Read the model definition and answer for the solid it produces. Units are mm, in the model's axes. A direction names the side the tool comes from. Coordinates: 2 decimals unless noted, no trailing zeros. Loops run counter-clockwise (first coordinate to the right, second up) from the corner with the lowest first, then second, coordinate; pieces in that order, holes last.
from build123d import *

# Parameters (mm, degrees)
F0_W     = 92.0124906
F0_H     = 21.3499954
F0_R     = 6.7062477
F1_DEPTH = 1.5875
F2_R     = 10.6749977
F4_DEPTH = 12
F5_R     = 2.2479
F6_DEPTH = 13.5875
F7_R     = 3.96875
F8_DEPTH = 7.2375014


with BuildPart() as f1:
    # F0 (on Top) → F1 (new body)
    with BuildSketch(Plane.XY):
        with Locations((46.0062453, -10.6749977)):
            Rectangle(F0_W, F0_H)
        with Locations((10.6749977, -10.6749977)):
            Circle(F0_R, mode=Mode.SUBTRACT)
        with Locations((81.3374929, -10.6749977)):
            Circle(F0_R, mode=Mode.SUBTRACT)
    extrude(amount=F1_DEPTH)

    # F2
    f2_edges = [f1.edges().sort_by_distance(p)[0] for p in [
        (0, 0, 0.79375),
        (92.012491, 0, 0.79375),
    ]]
    fillet(f2_edges, radius=F2_R)

    # F3 (on face) → F4 (join)
    with BuildSketch(Plane.XY.offset(1.5875)):
        with BuildLine():
            Line((4.5476495872, -14.9999954), (0, -14.9999954))
            Line((0, -14.9999954), (0, -21.3499954))
            Line((0, -21.3499954), (92.0124906, -21.3499954))
            Line((92.0124906, -21.3499954), (92.0124906, -14.9999954))
            Line((92.0124906, -14.9999954), (87.4648410128, -14.9999954))
            ThreePointArc((87.4648410128, -14.9999954), (81.3374929, -18.1749977), (75.2101447872, -14.9999954))
            Line((75.2101447872, -14.9999954), (16.8023458128, -14.9999954))
            ThreePointArc((16.8023458128, -14.9999954), (10.6749977, -18.1749977), (4.5476495872, -14.9999954))
        make_face()
        with BuildLine():
            Line((0, -10.6749977), (0, -14.9999954))
            Line((0, -14.9999954), (4.5476495872, -14.9999954))
            ThreePointArc((4.5476495872, -14.9999954), (8.4061996532, -3.5263925617), (18.1749977, -10.6749977))
            ThreePointArc((18.1749977, -10.6749977), (17.8236028383, -12.9437957468), (16.8023458128, -14.9999954))
            Line((16.8023458128, -14.9999954), (75.2101447872, -14.9999954))
            ThreePointArc((75.2101447872, -14.9999954), (79.0686948532, -3.5263925617), (88.8374929, -10.6749977))
            ThreePointArc((88.8374929, -10.6749977), (88.4860980383, -12.9437957468), (87.4648410128, -14.9999954))
            Line((87.4648410128, -14.9999954), (92.0124906, -14.9999954))
            Line((92.0124906, -14.9999954), (92.0124906, -10.6749977))
            ThreePointArc((92.0124906, -10.6749977), (88.8858561628, -3.1266344372), (81.3374929, 0))
            Line((81.3374929, 0), (10.6749977, 0))
            ThreePointArc((10.6749977, 0), (3.1266344372, -3.1266344372), (0, -10.6749977))
        make_face()
    extrude(amount=F4_DEPTH)

    # F5 (on face) → F6 (cut, through all)
    with BuildSketch(Plane.XY.offset(13.5875)):
        with Locations((25.3187477, -10.6749977)):
            Circle(F5_R)
        with Locations((66.6937429, -10.6749977)):
            Circle(F5_R)
        with BuildLine():
            ThreePointArc((46.0062453, -10.8706539), (48.2513093303, -9.9407179303), (49.1812453, -7.6956539))
            ThreePointArc((49.1812453, -7.6956539), (43.7611812697, -5.4505898697), (46.0062453, -10.8706539))
        make_face()
    extrude(amount=-F6_DEPTH, mode=Mode.SUBTRACT)

    # F7 (on face) → F8 (cut)
    with BuildSketch(Plane(origin=(0, 0, 0), x_dir=(1, 0, 0), z_dir=(0, 0, -1))):
        with Locations((66.6937429, 10.6749977)):
            Circle(F7_R)
        with Locations((25.3187477, 10.6749977)):
            Circle(F7_R)
    extrude(amount=-F8_DEPTH, mode=Mode.SUBTRACT)


solid = f1.part
Q1. Which of the six approach directions +Z, -Z, +X, -X, +Y, -Y give full straight-line access (tool end or side, diameter ignored) to faces 4 (the face through (68.4, -8.97, 7.238)), 5 (the face through (47, 0, 7)), 6 (the face through (5, -15, 1.588))?
Findings below:
face 4: -Z
face 5: +Z, -Z, +X, -X, +Y
face 6: +Z
Q2. A cutting plane is placed at D-D (x = 85). Give the vertices of the cut face in (y, z), then the cut area to 3 significant figures.
Findings below:
outline: (-21.35, 0) - (-16.29, 0) - (-16.29, 1.59) - (-17.22, 1.59) - (-17.22, 13.59) - (-21.35, 13.59) - close; (-5.06, 0) - (-0.65, 0) - (-0.65, 13.59) - (-4.13, 13.59) - (-4.13, 1.59) - (-5.06, 1.59) - close
area: 106 mm2
Q3. A cutting plane is placed at A-A (z = 3.5). Count the separate pieces of the cut face and the enclosed holes in it, then the cut area to 3 significant figures.
Findings below:
separate pieces: 1
enclosed holes: 5
area: 1,430 mm2
Q4. Determine the mould class of faces 1 (the face through (63.544, -8.26, 3.568)), 2 (the face through (45, -21.35, 7)), 3 (the face through (92.012, -16, 7)) for opening direction Y: +Y half, -Y half, draft (parallel to the pull), parting line (faces both ways), or undercut.
Findings below:
face 1: undercut
face 2: -Y half
face 3: draft
Q5. Flat-ended cylindrical pins translate along their axes: pin 1 Ø7 at (x, y) = (66.69, -10.67) entering from -Z; pin 2 Ø12 at (x, y) = (65, -14.5) entering from -Z; pin 3 Ø6 at (y, z) = (-5, 7.5) entering from -X. Find the tip coordinate at first contact, or state that the pin passes through.
Findings below:
pin 1: stops at z = 7.24
pin 2: stops at z = 0
pin 3: stops at x = 0.34
Q6. Straight lines are drawn through the part: probe 1 along X at (y, z) = (-7.75, 2); probe 2 along X at (y, z) = (-6, 13.25); probe 3 along X at (y, z) = (-15.25, 4). For each, find the intervals that lie inside material, in ascending order.
Findings below:
probe 1: x = 0.41 to 3.77, 17.58 to 22.64, 28 to 42.83, 49.18 to 64.01, 69.38 to 74.43, 88.24 to 91.6
probe 2: x = 1.08 to 4.81, 16.54 to 43.32, 48.69 to 75.47, 87.2 to 90.93
probe 3: x = 0 to 4.73, 16.62 to 75.39, 87.28 to 92.01
Q7. A cutting plane is placed at B-B (x = 47.5). Give the vertices of the cut face in (y, z).
Findings below:
outline: (-21.35, 0) - (-10.5, 0) - (-10.5, 13.59) - (-21.35, 13.59) - close; (-4.89, 0) - (0, 0) - (0, 13.59) - (-4.89, 13.59) - close
